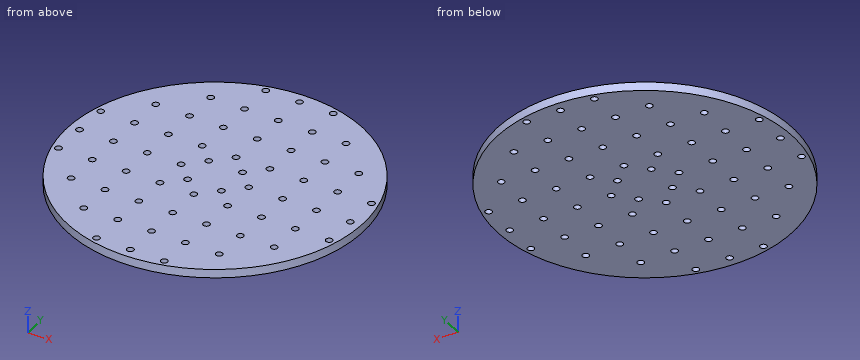
from build123d import *

# Parameters (mm, degrees)
SKETCH1_R           = 109.5375
SKETCH1_R_2         = 2.4892
BOSS_EXTRUDE1_DEPTH = 6.35
SKETCH2_R           = 2.4892
CUT_EXTRUDE1_DEPTH  = 6.35


with BuildPart() as part:
    # Sketch1 → Boss-Extrude1 (new body)
    with BuildSketch(Plane.XY):
        Circle(SKETCH1_R)
        with Locations((-12.7, 12.7)):
            Circle(SKETCH1_R_2, mode=Mode.SUBTRACT)
        with Locations((12.7, 12.7)):
            Circle(SKETCH1_R_2, mode=Mode.SUBTRACT)
        with Locations((12.7, -12.7)):
            Circle(SKETCH1_R_2, mode=Mode.SUBTRACT)
        with Locations((-12.7, -12.7)):
            Circle(SKETCH1_R_2, mode=Mode.SUBTRACT)
    extrude(amount=BOSS_EXTRUDE1_DEPTH)

    # Sketch2 → Cut-Extrude1 (cut)
    with BuildSketch(Plane.XY.offset(6.35)):
        with Locations((25.305046536, -101.6)):
            Circle(SKETCH2_R)
        with Locations((25.305046536, -76.2)):
            Circle(SKETCH2_R)
        with Locations((-76.294953464, 0)):
            Circle(SKETCH2_R)
        with Locations((-76.294953464, 25.4)):
            Circle(SKETCH2_R)
        with Locations((-76.294953464, 50.8)):
            Circle(SKETCH2_R)
        with Locations((-0.094953464, -76.2)):
            Circle(SKETCH2_R)
        with Locations((50.705046536, -76.2)):
            Circle(SKETCH2_R)
        with Locations((-25.494953464, -50.8)):
            Circle(SKETCH2_R)
        with Locations((-0.094953464, -50.8)):
            Circle(SKETCH2_R)
        with Locations((25.305046536, -50.8)):
            Circle(SKETCH2_R)
        with Locations((50.705046536, -50.8)):
            Circle(SKETCH2_R)
        with Locations((76.105046536, -50.8)):
            Circle(SKETCH2_R)
        with Locations((-50.894953464, -25.4)):
            Circle(SKETCH2_R)
        with Locations((-25.494953464, -25.4)):
            Circle(SKETCH2_R)
        with Locations((-0.094953464, -25.4)):
            Circle(SKETCH2_R)
        with Locations((25.305046536, -25.4)):
            Circle(SKETCH2_R)
        with Locations((50.705046536, -25.4)):
            Circle(SKETCH2_R)
        with Locations((76.105046536, -25.4)):
            Circle(SKETCH2_R)
        with Locations((101.505046536, -25.4)):
            Circle(SKETCH2_R)
        with Locations((-50.894953464, 0)):
            Circle(SKETCH2_R)
        with Locations((-25.494953464, 0)):
            Circle(SKETCH2_R)
        with Locations((25.305046536, 0)):
            Circle(SKETCH2_R)
        with Locations((50.705046536, 0)):
            Circle(SKETCH2_R)
        with Locations((76.105046536, 0)):
            Circle(SKETCH2_R)
        with Locations((101.505046536, 0)):
            Circle(SKETCH2_R)
        with Locations((-50.894953464, 25.4)):
            Circle(SKETCH2_R)
        with Locations((-25.494953464, 25.4)):
            Circle(SKETCH2_R)
        with Locations((-0.094953464, 25.4)):
            Circle(SKETCH2_R)
        with Locations((25.305046536, 25.4)):
            Circle(SKETCH2_R)
        with Locations((50.705046536, 25.4)):
            Circle(SKETCH2_R)
        with Locations((76.105046536, 25.4)):
            Circle(SKETCH2_R)
        with Locations((101.505046536, 25.4)):
            Circle(SKETCH2_R)
        with Locations((-50.894953464, 50.8)):
            Circle(SKETCH2_R)
        with Locations((-25.494953464, 50.8)):
            Circle(SKETCH2_R)
        with Locations((-0.094953464, 50.8)):
            Circle(SKETCH2_R)
        with Locations((25.305046536, 50.8)):
            Circle(SKETCH2_R)
        with Locations((50.705046536, 50.8)):
            Circle(SKETCH2_R)
        with Locations((76.105046536, 50.8)):
            Circle(SKETCH2_R)
        with Locations((-50.894953464, 76.2)):
            Circle(SKETCH2_R)
        with Locations((-25.494953464, 76.2)):
            Circle(SKETCH2_R)
        with Locations((-0.094953464, 76.2)):
            Circle(SKETCH2_R)
        with Locations((25.305046536, 76.2)):
            Circle(SKETCH2_R)
        with Locations((50.705046536, 76.2)):
            Circle(SKETCH2_R)
        with Locations((-25.494953464, 101.6)):
            Circle(SKETCH2_R)
        with Locations((-0.094953464, 101.6)):
            Circle(SKETCH2_R)
        with Locations((25.305046536, 101.6)):
            Circle(SKETCH2_R)
        with Locations((-25.494953464, -101.6)):
            Circle(SKETCH2_R)
        with Locations((-0.094953464, -101.6)):
            Circle(SKETCH2_R)
        with Locations((-50.894953464, -76.2)):
            Circle(SKETCH2_R)
        with Locations((-25.494953464, -76.2)):
            Circle(SKETCH2_R)
        with Locations((-76.294953464, -50.8)):
            Circle(SKETCH2_R)
        with Locations((-50.894953464, -50.8)):
            Circle(SKETCH2_R)
        with Locations((-76.294953464, -25.4)):
            Circle(SKETCH2_R)
        with Locations((-101.694953464, -25.4)):
            Circle(SKETCH2_R)
        with Locations((-101.694953464, 0)):
            Circle(SKETCH2_R)
        with Locations((-101.694953464, 25.4)):
            Circle(SKETCH2_R)
    extrude(amount=-CUT_EXTRUDE1_DEPTH, mode=Mode.SUBTRACT)


solid = part.part
Work out the finished part from the listing and answer in its coordinate system (mm). Round coordinates to 2 decimals unless told otherwise and drop trailing zeros. Loops run counter-clockwise (first coordinate to the right, second up) from the corner with the lowest first, then second, coordinate; pieces in that order, holes last. Notation, with made-up numbers: (87, 17) - (111, 17) arc R12 cw to (111, 24) - close; hole circle Ø2 at (-40, 22.25). An arc over 180 degrees is marked (long way). Use one line per item in the form item = value. Start each with the question number.
(1) Consider line 1 (Y direction, x = -11.5, z = 4.5); line 2 (Y direction, x = -12.7, z = 3.5); line 3 (X direction, y = 34, z = 0.5). Determine where each line is inside the solid, lowest interval first.
(2) Flat-ended cylindrical pins translate along their axes: P1, Ø8, axis at x = -25.49, y = -76.2, coming from the -Z side; P2, Ø3, axis at y = -71, z = 4.5, coming from the -X side; P3, Ø4, axis at x = -0.09, y = -25.4, coming from the -Z side; P4, Ø1, axis at y = 16.5, z = 4, coming from the -X side. Find the tip coordinate at first contact, or state that the pin passes through.
(3) Find section B-B on x = 12.7. Determine the outline of the cut face in (y, z), and give its area (3 significant figures).
(4) Find section D-D on y = 76.2. Determine the outline of the cut face in (x, z).
(5) Find section A-A on y = 50.8. Give the number of separate pieces and of enclosed holes in the cut face, and give its area (3 significant figures).
Answer list:
q1.line_1 = -108.93 to -14.88, -10.52 to 10.52, 14.88 to 108.93
q1.line_2 = -108.8 to -15.19, -10.21 to 10.21, 15.19 to 108.8
q1.line_3 = -104.13 to 104.13
q2.P1 = 0
q2.P2 = -84.67
q2.P3 = through
q2.P4 = -108.36
q3.outline = (-108.8, 0) - (-15.19, 0) - (-15.19, 6.35) - (-108.8, 6.35) - close; (-10.21, 0) - (10.21, 0) - (10.21, 6.35) - (-10.21, 6.35) - close; (15.19, 0) - (108.8, 0) - (108.8, 6.35) - (15.19, 6.35) - close
q3.area = 1,320 mm^2
q4.outline = (-78.69, 0) - (-53.38, 0) - (-53.38, 6.35) - (-78.69, 6.35) - close; (-48.41, 0) - (-27.98, 0) - (-27.98, 6.35) - (-48.41, 6.35) - close; (-23.01, 0) - (-2.58, 0) - (-2.58, 6.35) - (-23.01, 6.35) - close; (2.39, 0) - (22.82, 0) - (22.82, 6.35) - (2.39, 6.35) - close; (27.79, 0) - (48.22, 0) - (48.22, 6.35) - (27.79, 6.35) - close; (53.19, 0) - (78.69, 0) - (78.69, 6.35) - (53.19, 6.35) - close
q5.separate_pieces = 8
q5.enclosed_holes = 0
q5.area = 1,010 mm^2
